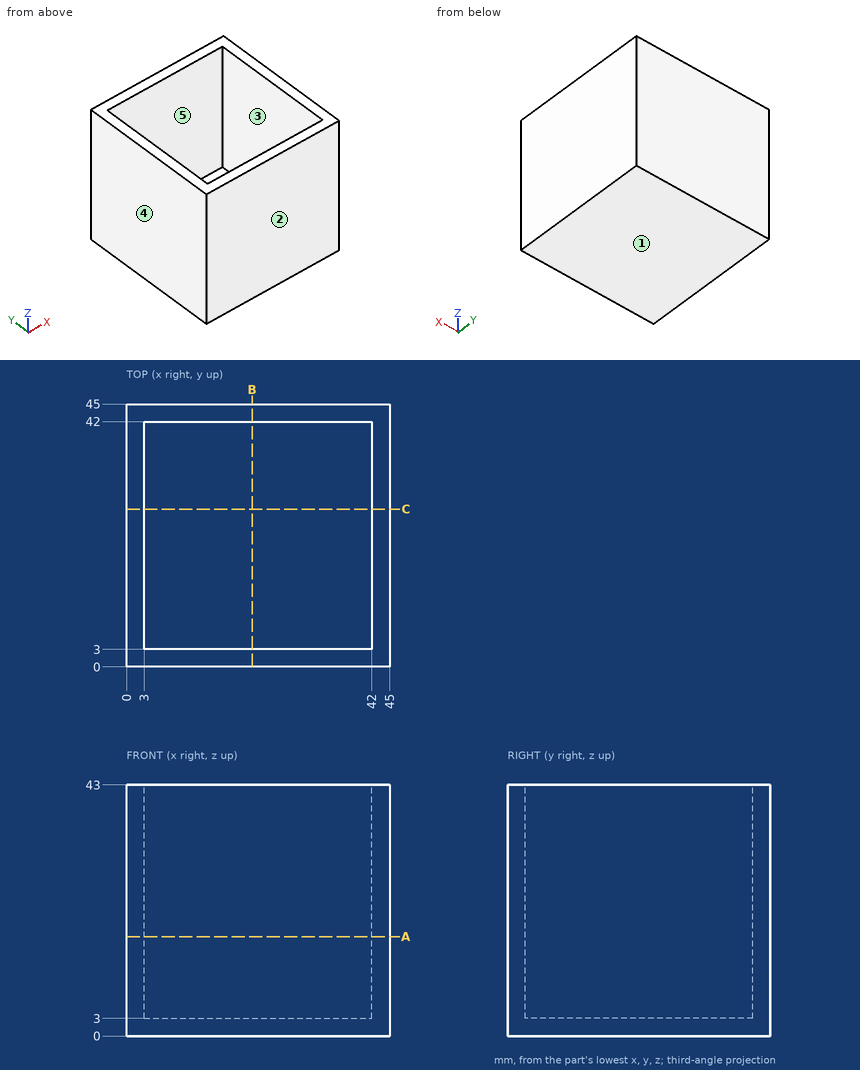
Can you work these out from the drawing? Everything is in mm from the part's minimum corner. A direction names the side the tool comes from. Round coordinates to 2 decimals unless told otherwise and drop trailing zeros. Write each loop counter-clockwise with the first axis right and the second up, starting at its lowest first coordinate (ties: lowest second). Pieces come first, ordered by that corner, then holes.
1. Suppose I cut it at A-A (z = 17). List the corners of the cut face in (x, y) for me, and give its area (3 significant figures).
2. Will these pins go through, and if not, where does the flat tip stop? pin 1 Ø1.5 at (x, y) = (29.5, 5) entering from +Z; pin 2 Ø1 at (x, z) = (33, 33) entering from -Y.
3. For the marked faces 4 and 5, which set-ups out of +Z, -Z, +X, -X, +Y, -Y let a thin tool reach every point of the face, with its end or its side?
4. If we mould it in two halves opening along Y, with no side actions, what happens to the marked faces 1, 2 and 3? For each: released by +Y, released by -Y, zero draft, split by the parting line, or undercut.
5. I need wall thicknesses on L1, parallel to X at y = 37, z = 15; L2, parallel to Z at x = 39, y = 21. Which ranges of each line are inside material? Lowest first, please.
6. Suppose I cut it at B-B (x = 21.5). List the corners of the cut face in (y, z) for me, and give its area (3 significant figures).
Answer sheet:
1. outline: (0, 0) - (45, 0) - (45, 45) - (0, 45) - close; hole (3, 3) - (42, 3) - (42, 42) - (3, 42) - close
1. area: 504 mm2
2. pin 1: stops at z = 3
2. pin 2: stops at y = 0
3. face 4: +Z, -Z, -X, +Y, -Y
3. face 5: +Z
4. face 1: zero draft
4. face 2: released by -Y
4. face 3: undercut
5. L1: x = 0 to 3, 42 to 45
5. L2: z = 0 to 3
6. outline: (0, 0) - (45, 0) - (45, 43) - (42, 43) - (42, 3) - (3, 3) - (3, 43) - (0, 43) - close
6. area: 375 mm2
